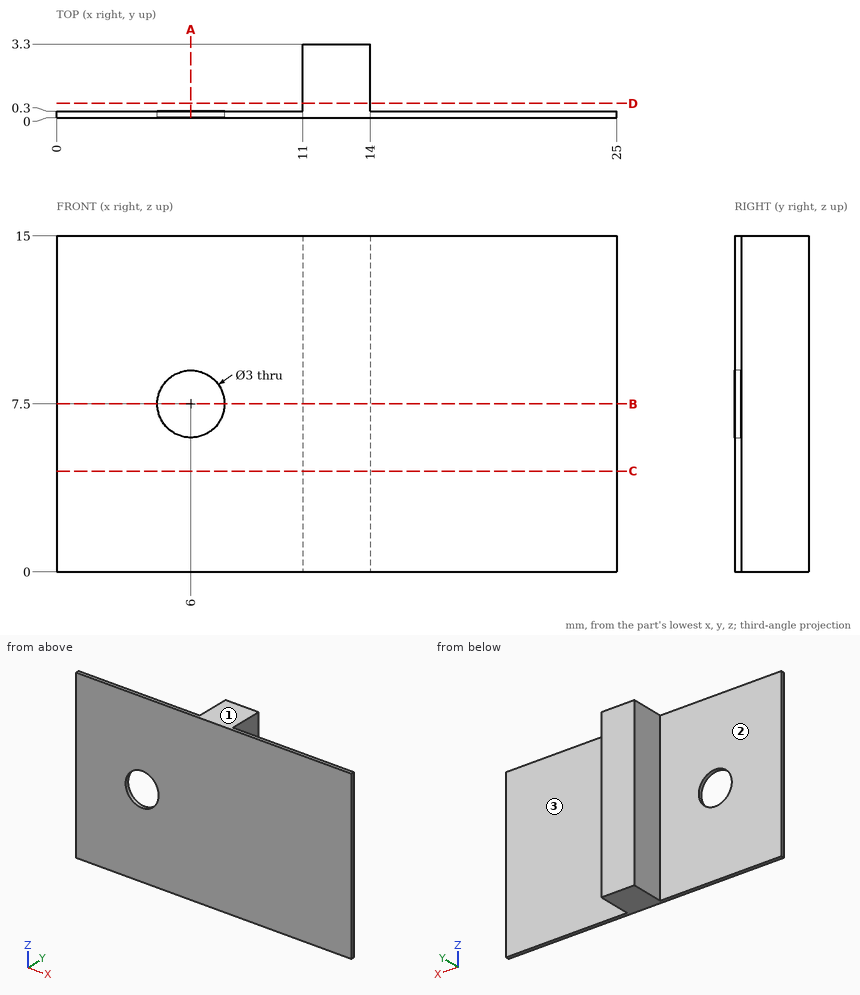
The drawing under review shows one solid part. Ordinate dimensions are in mm from its lowest x, y, z. A direction names the side the tool comes from. Round coordinates to 2 decimals unless told otherwise and drop trailing zeros. Order: outer loops, then holes, each group sorted by start corner. A loop starts at its lowest first (then second) coordinate and runs counter-clockwise, first axis right, second up. Notation, with made-up numbers: (80.5, 70) -> (91.5, 70) arc R16 cw to (91.5, 98) -> close; hole circle Ø5 at (-5.5, 4). An arc over 180 degrees is marked (long way). Return JSON: item names as keys, results as strings.
1. Take a section at D-D (y = 0.65). Write out the cut boundary in (x, z), then the cut area to 3 significant figures.
Answer block:
{"outline": "(11, 0) -> (14, 0) -> (14, 15) -> (11, 15) -> close", "area": "45.0 mm²"}
2. Take a section at C-C (z = 4.5). Write out the cut boundary in (x, y), then the cut area to 3 significant figures.
Answer block:
{"outline": "(0, 0) -> (25, 0) -> (25, 0.3) -> (14, 0.3) -> (14, 3.3) -> (11, 3.3) -> (11, 0.3) -> (0, 0.3) -> close", "area": "16.5 mm²"}
3. Insertion check: P1, Ø9, axis at x = 5.5, z = 6.5, coming from the +Y side. The pin has a flat end and moves straight along its axis. Give the tip position at first contact, or say it passes through.
Answer block:
{"P1": "stops at y = 0.3"}
4. Take a section at A-A (x = 6). Write out the cut boundary in (y, z), then the cut area to 3 significant figures.
Answer block:
{"outline": "(0, 0) -> (0.3, 0) -> (0.3, 6) -> (0, 6) -> close; (0, 9) -> (0.3, 9) -> (0.3, 15) -> (0, 15) -> close", "area": "3.60 mm²"}
5. For the marked faces 1, 2 and 3, list the 3-axis set-ups (+Z, -Z, +X, -X, +Y, -Y) from which the entire face can be reached by the end or side of a thin tool; tool diameter is ignored.
Answer block:
{"face 1": "+Z, +X, -X, +Y, -Y", "face 2": "+Z, -Z, -X, +Y", "face 3": "+Z, -Z, +X, +Y"}
6. Take a section at B-B (z = 7.5). Write out the cut boundary in (x, y), then the cut area to 3 significant figures.
Answer block:
{"outline": "(0, 0) -> (4.5, 0) -> (4.5, 0.3) -> (0, 0.3) -> close; (7.5, 0) -> (25, 0) -> (25, 0.3) -> (14, 0.3) -> (14, 3.3) -> (11, 3.3) -> (11, 0.3) -> (7.5, 0.3) -> close", "area": "15.6 mm²"}
7. For L1, parallel to X at y = 0.25, z = 7.5; L2, parallel to X at y = 1.2, z = 6.5; L3, parallel to Y at x = 8, z = 12.25, list the stretches that pass through material, from the lowest coordinate up. Write a range as [from, to].
Answer block:
{"L1": "x = [0, 4.5], [7.5, 25]", "L2": "x = [11, 14]", "L3": "y = [0, 0.3]"}
